from build123d import *

# Parameters (mm, degrees)
F1_DEPTH = 2
F3_DEPTH = 2
F5_DEPTH = 2
F6_R     = 1.75
F7_DEPTH = 6


with BuildPart() as f1:
    # F0 (on Front) → F1 (new body)
    with BuildSketch(Plane.XZ):
        with BuildLine():
            Line((36.0155949142, 4.5501915368), (34.5935707333, 3.7231953967))
            ThreePointArc((34.5935707333, 3.7231953967), (34.4002745916, 3.51961513), (34.3471502153, 3.2439593227))
            ThreePointArc((34.3471502153, 3.2439593227), (34.4617663682, 1.6237791679), (34.5, 0))
            ThreePointArc((34.5, 0), (33.5, -1), (32.5, 0))
            ThreePointArc((32.5, 0), (32.4611135591, 1.589372991), (32.344547292, 3.1749425938))
            ThreePointArc((32.344547292, 3.1749425938), (32.3418598815, 3.4374174131), (32.3849685604, 3.6963419093))
            Line((32.3849685604, 3.6963419093), (34.5683472951, 12.1558157161))
            ThreePointArc((34.5683472951, 12.1558157161), (34.6283647637, 12.7729522849), (34.4964834196, 13.3788127905))
            ThreePointArc((34.4964834196, 13.3788127905), (-7.3396727546, 36.2647101719), (-36.9839930773, -1.0882352941))
            ThreePointArc((-36.9839930773, -1.0882352941), (-36.075182574, -3.1522901619), (-33.9852909359, -4))
            Line((-33.9852909359, -4), (-29.7321374946, -4))
            Line((-29.7321374946, -4), (0, -4))
            ThreePointArc((0, -4), (4, 0), (0, 4))
            Line((0, 4), (-27.3495886624, 4))
            ThreePointArc((-27.3495886624, 4), (-28.9079761073, 4.7464336589), (-29.3031307097, 6.4285714286))
            ThreePointArc((-29.3031307097, 6.4285714286), (3.2331160442, 29.825273857), (30, 0))
            ThreePointArc((30, 0), (33.5, -3.5), (37, 0))
            ThreePointArc((37, 0), (36.9408945016, 2.0905294604), (36.7637668419, 4.1743799053))
            ThreePointArc((36.7637668419, 4.1743799053), (36.4913900405, 4.5647699812), (36.0155949142, 4.5501915368))
        make_face()
    extrude(amount=F1_DEPTH)

    # F2 (on face) → F3 (join)
    with BuildSketch(Plane.XZ.offset(2)):
        with BuildLine():
            ThreePointArc((0, -4), (2.8284271247, -2.8284271247), (4, 0))
            ThreePointArc((4, 0), (2.8284271247, 2.8284271247), (0, 4))
            ThreePointArc((0, 4), (-4, 0), (0, -4))
        make_face()
    extrude(amount=F3_DEPTH)

    # F4 (on face) → F5 (join)
    with BuildSketch(Plane.XZ.offset(4)):
        with BuildLine():
            Line((36.0155949142, 4.5501915368), (34.5935707333, 3.7231953967))
            ThreePointArc((34.5935707333, 3.7231953967), (34.4002745916, 3.51961513), (34.3471502153, 3.2439593227))
            ThreePointArc((34.3471502153, 3.2439593227), (34.4617663682, 1.6237791679), (34.5, 0))
            ThreePointArc((34.5, 0), (33.5, -1), (32.5, 0))
            ThreePointArc((32.5, 0), (32.4611135591, 1.589372991), (32.344547292, 3.1749425938))
            ThreePointArc((32.344547292, 3.1749425938), (32.3418598815, 3.4374174131), (32.3849685604, 3.6963419093))
            Line((32.3849685604, 3.6963419093), (34.5683472951, 12.1558157161))
            ThreePointArc((34.5683472951, 12.1558157161), (34.6283647637, 12.7729522849), (34.4964834196, 13.3788127905))
            ThreePointArc((34.4964834196, 13.3788127905), (-7.3396727546, 36.2647101719), (-36.9839930773, -1.0882352941))
            ThreePointArc((-36.9839930773, -1.0882352941), (-36.075182574, -3.1522901619), (-33.9852909359, -4))
            Line((-33.9852909359, -4), (-29.7321374946, -4))
            Line((-29.7321374946, -4), (0, -4))
            ThreePointArc((0, -4), (-4, 0), (0, 4))
            Line((0, 4), (-27.3495886624, 4))
            ThreePointArc((-27.3495886624, 4), (-28.9079761073, 4.7464336589), (-29.3031307097, 6.4285714286))
            ThreePointArc((-29.3031307097, 6.4285714286), (3.2331160442, 29.825273857), (30, 0))
            ThreePointArc((30, 0), (33.5, -3.5), (37, 0))
            ThreePointArc((37, 0), (36.9408945016, 2.0905294604), (36.7637668419, 4.1743799053))
            ThreePointArc((36.7637668419, 4.1743799053), (36.4913900405, 4.5647699812), (36.0155949142, 4.5501915368))
        make_face()
        with BuildLine():
            ThreePointArc((4, 0), (2.8284271247, 2.8284271247), (0, 4))
            ThreePointArc((0, 4), (-4, 0), (0, -4))
            ThreePointArc((0, -4), (2.8284271247, -2.8284271247), (4, 0))
        make_face()
    extrude(amount=F5_DEPTH)

    # F6 (on face) → F7 (cut)
    with BuildSketch(Plane(origin=(0, 0, 0), x_dir=(-1, 0, 0), z_dir=(0, 1, 0))):
        Circle(F6_R)
    extrude(amount=-F7_DEPTH, mode=Mode.SUBTRACT)


solid = f1.part
Verification items for the finished model (mm, model axes). A direction names the side the tool comes from. Give positions to 0.01 mm unless a question says otherwise; leave off trailing zeros. Write each loop counter-clockwise with the first axis right and the second up, starting at its lowest first coordinate (ties: lowest second). Pieces come first, ordered by that corner, then holes. Notation, with made-up numbers: (16, 27.25) - (23, 27.25) arc R16 ccw to (23, 36.25) - close; hole circle Ø1 at (49, 6). An arc over 180 degrees is marked (long way). Answer as CSV lines item,"result". Start each with the question number.
1. Draft check along Y on faces 1 (the face through (3.966, -2.958, 0.521)), 2 (the face through (35.31, -0.99, 4.14)), 3 (the face through (-9, -6, 3)). Enter one of: pulls with the +Y half, pulls with the -Y half, needs draft (parallel to the pull), parting line crosses it, or undercut.
2. Sectioned sample at A-A (y = -5). Record the boundary of the cut face in (x, z).
3. Sectioned sample at D-D (x = 33.5). Record the boundary of the cut face in (y, z), then the cut area to 3 significant figures.
4. Sectioned sample at C-C (x = -32). Record the boundary of the cut face in (y, z), then the cut area to 3 significant figures.
5. Set-up check for faces 4 (the face through (-36.1, -0.99, -3.13)), 5 (the face through (34.46, -0.99, 1.65)): record each of +Z, -Z, +X, -X, +Y, -Y from which the full face is reachable in a straight line by a thin tool's end or side.
6. Sectioned sample at B-B (z = 25). Record the boundary of the cut face in (x, y).
7. Thickness scan on line 1 (Y direction, x = -8, z = 32); line 2 (Z direction, x = 0, y = -2.65); line 3 (X direction, y = -5, z = 16). Record the ranges inside material, lowest first.
8. Depth check by flat-ended pin: pin 1 (2 mm diameter, centred on x = -16.5, y = -0.5, fed in from +Z); pin 2 (1.5 mm diameter, centred on y = -3, z = 11.5, fed in from +X); pin 3 (1.5 mm diameter, centred on y = -5, z = 2, fed in from -X); pin 4 (3 mm diameter, centred on y = -2.5, z = 15, fed in from -X). Enter the tip coordinate at first touch or a pass-through.
Derived:
1,face 1,"undercut"
1,face 2,"needs draft"
1,face 3,"pulls with the -Y half"
2,outline,"(-36.98, -1.09) arc R3 ccw to (-33.99, -4) - (0, -4) arc R4 ccw to (0, 4) - (-27.35, 4) arc R2 cw to (-29.3, 6.43) arc R30 cw to (30, 0) arc R3.5 ccw to (37, 0) arc R37 ccw to (36.76, 4.17) arc R0.5 ccw to (36.02, 4.55) - (34.59, 3.72) arc R0.5 ccw to (34.35, 3.24) arc R34.5 cw to (34.5, 0) arc R1 cw to (32.5, 0) arc R32.5 ccw to (32.34, 3.17) arc R1.5 cw to (32.38, 3.7) - (34.57, 12.16) arc R2 ccw to (34.5, 13.38) arc R37 ccw to start; hole circle Ø3.5 at (0, 0)"
3,outline,"(-6, -3.5) - (-4, -3.5) - (-4, -1) - (-6, -1) - close; (-6, 8.02) - (-4, 8.02) - (-4, 15.71) - (-6, 15.71) - close; (-2, -3.5) - (0, -3.5) - (0, -1) - (-2, -1) - close; (-2, 8.02) - (0, 8.02) - (0, 15.71) - (-2, 15.71) - close"
3,area,"40.8 mm²"
4,outline,"(-6, -4) - (-4, -4) - (-4, 18.57) - (-6, 18.57) - close; (-2, -4) - (0, -4) - (0, 18.57) - (-2, 18.57) - close"
4,area,"90.3 mm²"
5,face 4,"-Z, -X, +Y, -Y"
5,face 5,"+Y, -Y"
6,outline,"(-27.28, -6) - (-16.58, -6) - (-16.58, -4) - (-27.28, -4) - close; (-27.28, -2) - (-16.58, -2) - (-16.58, 0) - (-27.28, 0) - close; (16.58, -6) - (27.28, -6) - (27.28, -4) - (16.58, -4) - close; (16.58, -2) - (27.28, -2) - (27.28, 0) - (16.58, 0) - close"
7,line 1,"-6 to -4, -2 to 0"
7,line 2,"-4 to -1.75, 1.75 to 4"
7,line 3,"-33.36 to -25.38, 25.38 to 33.36"
8,pin 1,"z = 33.6"
8,pin 2,"through"
8,pin 3,"x = -36.98"
8,pin 4,"x = -34.42"
